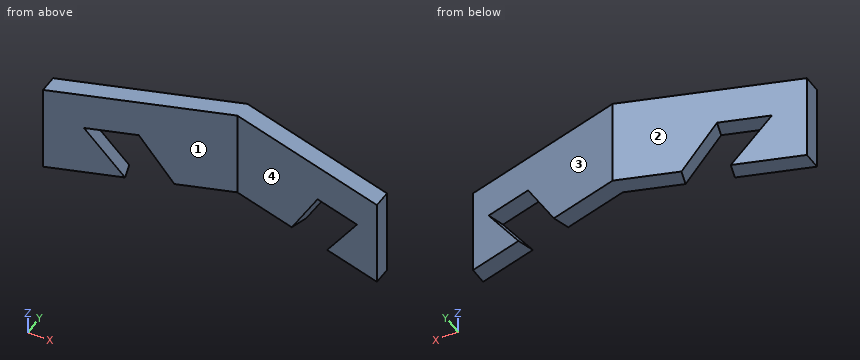
from build123d import *

# Parameters (mm, degrees)
F1_DEPTH = 25.4
F3_DEPTH = 33.2294348111
F5_DEPTH = 19.1997730291
F7_DEPTH = 33.2294348111


with BuildPart() as f1:
    # F0 (on Top) → F1 (new body)
    with BuildSketch(Plane.XY):
        Polygon((-48.6410071966, 22.7927347302), (0, 37.4451208464), (0, 42.8436696529), (-48.6410071966, 28.1912835367), align=None)
        Polygon((0, 42.8436696529), (0, 37.4451208464), (48.6410071966, 22.7927347302), (48.6410071966, 28.1912835367), align=None)
    extrude(amount=F1_DEPTH)

    # F2 (on face) → F3 (cut, through all)
    with BuildSketch(Plane(origin=(-11.8323266679, 39.2793557338, 0), x_dir=(-0.9575001417, -0.2884327976, 0), z_dir=(-0.2884327976, 0.9575001417, 0))):
        Polygon((5.6493859738, 0), (18.5344964266, 0), (29.307289049, 14.6010806784), (14.9435615167, 14.6010806784), align=None)
    extrude(amount=-F3_DEPTH, mode=Mode.SUBTRACT)

    # F4 (on face) → F5 (cut, through all)
    with BuildSketch(Plane(origin=(10.34138545, 34.3299309825, 0), x_dir=(0.9575001417, -0.2884327976, 0), z_dir=(-0.2884327976, -0.9575001417, 0))):
        Polygon((9.0973575134, 0.1226081513), (21.9824679662, 0.1226081513), (32.7552605886, 14.7236888297), (18.3915330563, 14.7236888297), align=None)
    extrude(amount=-F5_DEPTH, mode=Mode.SUBTRACT)

    # F6 (on face) → F7 (cut, through all)
    with BuildSketch(Plane(origin=(11.8323266679, 39.2793557338, 0), x_dir=(-0.9575001417, 0.2884327976, 0), z_dir=(0.2884327976, 0.9575001417, 0))):
        Polygon((-12.5681698828, 5.5752285791), (-25.2396277855, 4.5372529859), (-17.4372941709, -6.037767492), (-5.5907663486, -5.3862204982), align=None)
    extrude(amount=-F7_DEPTH, mode=Mode.SUBTRACT)


solid = f1.part
Source: CAD feature listing. Evaluate the final solid. Frame: model axes, mm. Face numbers are marked on the shaded views. Give positions to 0.01 mm unless a question says otherwise; leave off trailing zeros. Loops run counter-clockwise (first coordinate to the right, second up) from the corner with the lowest first, then second, coordinate; pieces in that order, holes last. Notation, with made-up numbers: (49, 73) -> (72, 73) arc R18 cw to (72, 105) -> close; hole circle Ø5 at (63, 55.25). An arc over 180 degrees is marked (long way). Use a Markdown table: item, result. Add a question column.
1) Line query: line 1 along X through (y, z) = (27.5, 7.25); line 2 along Y through (x, z) = (-33.5, 3.75); line 3 along Y through (x, z) = (36, 23.5). Output: solid intervals per line, ascending. Write a range as [from, to].
2) Section query D-D, the plane z = 12.75. Return the cut outline in (x, y).
3) Section query C-C, the plane z = 17.25. Return the cut outline in (x, y).
4) First-contact query: pin 1 (8 mm diameter, centred on x = -4.5, z = 22, fed in from -Y); pin 2 (3 mm diameter, centred on x = -4.5, z = 20.5, fed in from -Y); pin 3 (1.5 mm diameter, centred on x = -1.5, z = 21.5, fed in from -Y). Flat tips, straight axial feed; report the tip coordinate or a pass-through.
5) Pull-direction query (X, two-part tool) for the marked faces 1, 2, 3 and 4; classes: +X half, -X half, draft (parallel to the pull), parting line (faces both ways), or undercut.
6) Section query B-B, the plane z = 5.75. Return the cut outline in (x, y), then the cut area to 3 significant figures.
7) Section query A-A, the plane x = 36.5. Return the cut outline in (y, z).
Numbers:
| question | item | result |
|---|---|---|
| 1 | line 1 | x = [-48.64, -33.23], [36.73, 48.64] |
| 1 | line 2 | y = [27.35, 32.75] |
| 1 | line 3 | y = [26.6, 32] |
| 2 | outline | (-48.64, 22.79) -> (-37.1, 26.27) -> (-38.59, 31.22) -> (-48.64, 28.19) -> close; (-25.01, 35.31) -> (-23.52, 30.36) -> (0, 37.45) -> (26.75, 29.39) -> (28.24, 34.34) -> (0, 42.84) -> close; (40.31, 25.3) -> (48.64, 22.79) -> (48.64, 28.19) -> (41.8, 30.25) -> close |
| 3 | outline | (-48.64, 22.79) -> (0, 37.45) -> (48.64, 22.79) -> (48.64, 28.19) -> (0, 42.84) -> (-48.64, 28.19) -> close |
| 4 | pin 1 | stops at y = 34.88 |
| 4 | pin 2 | stops at y = 35.64 |
| 4 | pin 3 | stops at y = 36.77 |
| 5 | face 1 | undercut |
| 5 | face 2 | -X half |
| 5 | face 3 | +X half |
| 5 | face 4 | undercut |
| 6 | outline | (-48.64, 22.79) -> (-32.15, 27.76) -> (-33.64, 32.71) -> (-48.64, 28.19) -> close; (-20.75, 36.59) -> (-19.26, 31.64) -> (0, 37.45) -> (22.48, 30.67) -> (23.97, 35.62) -> (0, 42.84) -> close; (35.37, 26.79) -> (48.64, 22.79) -> (48.64, 28.19) -> (36.86, 31.74) -> close |
| 6 | area | 386 mm2 |
| 7 | outline | (26.45, 0) -> (31.85, 0) -> (31.85, 5.25) -> (26.45, 7.36) -> close; (26.45, 14.72) -> (31.85, 14.72) -> (31.85, 25.4) -> (26.45, 25.4) -> close |
